Verification items for the finished model (mm, model axes). Coordinates: 2 decimals unless noted, no trailing zeros. Write each loop counter-clockwise with the first axis right and the second up, starting at its lowest first coordinate (ties: lowest second). Pieces come first, ordered by that corner, then holes. Notation, with made-up numbers: (75.5, 32.5) -> (109.5, 32.5) arc R14 cw to (109.5, 42.5) -> close; hole circle Ø6 at (-6.75, 83.25). An arc over 180 degrees is marked (long way). Answer in a Markdown table with one row per item.
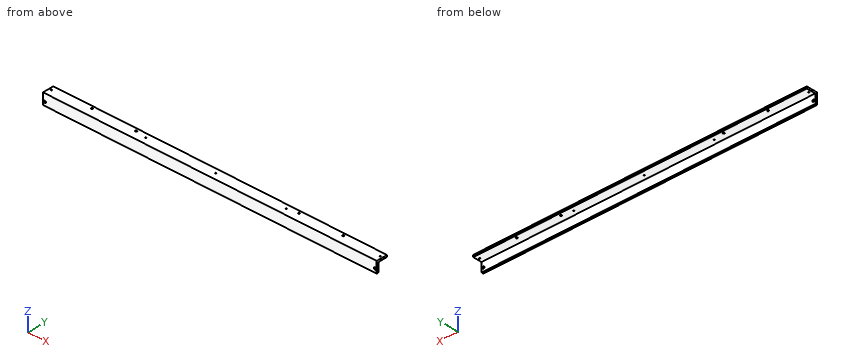
```python
from build123d import *

# Parameters (mm, degrees)
EXTRUDE1_DEPTH          = 573.0875
F_1_4_CLEARANCE_HOLE1_D = 7.14248
F_10_24_TAPPED_HOLE1_D  = 3.7973
F_10_CLEARANCE_HOLE1_D  = 5.6134


with BuildPart() as part:
    # Sketch1 → Extrude1 (new, symmetric)
    with BuildSketch(Plane(origin=(0, 0, 0), x_dir=(0, 0, -1), z_dir=(1, 0, 0))):
        with BuildLine():
            Line((0, 38.1), (0, 0))
            Line((0, 0), (38.1, 0))
            Line((38.1, 0), (38.1, 4.826))
            ThreePointArc((38.1, 4.826), (37.653630735, 5.903630735), (36.576, 6.35))
            Line((36.576, 6.35), (6.35, 6.35))
            Line((6.35, 6.35), (6.35, 36.576))
            ThreePointArc((6.35, 36.576), (5.903630735, 37.653630735), (4.826, 38.1))
            Line((4.826, 38.1), (0, 38.1))
        make_face()
    extrude(amount=EXTRUDE1_DEPTH, both=True)

    # 1/4 Clearance Hole1 (through all)
    with Locations(Plane(origin=(0, 6.35, 0), x_dir=(-1, 0, 0), z_dir=(0, 1, 0))):
        with Locations((-566.7375, -25.4), (566.7375, -25.4)):
            Hole(F_1_4_CLEARANCE_HOLE1_D / 2)

    # #10-24 Tapped Hole1 (through all)
    with Locations(Plane.XY):
        with Locations((-565.15, 22.225), (565.15, 22.225), (-241.3, 22.225), (241.3, 22.225), (0, 22.225)):
            Hole(F_10_24_TAPPED_HOLE1_D / 2)

    # #10 Clearance Hole1 (through all)
    with Locations(Plane.XY):
        with Locations((-431.8, 28.575), (-279.4, 28.575), (279.4, 28.575), (431.8, 28.575)):
            Hole(F_10_CLEARANCE_HOLE1_D / 2)


solid = part.part
```
1. Thickness scan on line 1 (Z direction, x = -271, y = 17); line 2 (Y direction, x = -232.5, z = -16.5); line 3 (Y direction, x = 0, z = -4.25). Record the ranges inside material, lowest first. Write a range as from..to.
Geometry says:
| item | result |
|---|---|
| line 1 | -6.35..0 |
| line 2 | 0..6.35 |
| line 3 | 0..20.33, 24.12..38.1 |
2. Section check A-A, the plane x = -81.5. Record the boundary of the cut face in (y, z).
Geometry says:
| item | result |
|---|---|
| outline | (0, -38.1) -> (4.83, -38.1) arc R1.52 ccw to (6.35, -36.58) -> (6.35, -6.35) -> (36.58, -6.35) arc R1.52 ccw to (38.1, -4.83) -> (38.1, 0) -> (0, 0) -> close |
3. Depth check by flat-ended pin: P1, Ø5, axis at x = 565.15, y = 22.225, coming from the -Z side; P2, Ø15, axis at x = 116.5, z = -26.5, coming from the +Y side. Enter the tip coordinate at first touch or a pass-through.
Geometry says:
| item | result |
|---|---|
| P1 | z = -6.35 |
| P2 | y = 6.35 |
